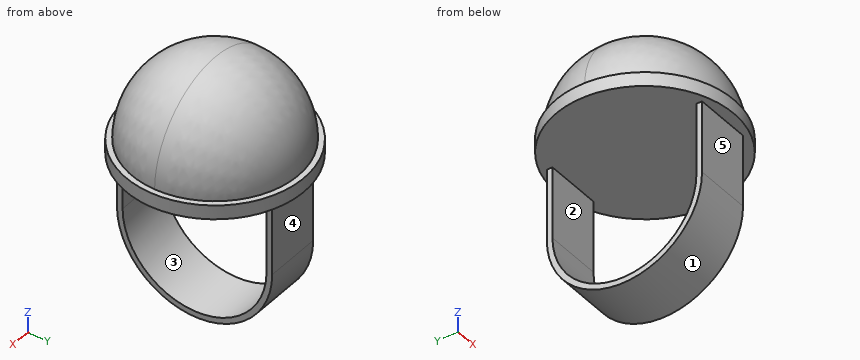
from build123d import *

# Parameters (mm, degrees)
F1_ANGLE = 180
F2_R     = 31.5
F3_DEPTH = 5
F4_W     = 20
F4_H     = 2
F5_DEPTH = 25.5
F6_W     = 20
F6_H     = 2
F7_ANGLE = 180


with BuildPart() as f1:
    # F0 (on Top) → F1 (revolve)
    with BuildSketch(Plane.XY):
        with BuildLine():
            ThreePointArc((0, -29.5), (20.85965, -20.85965), (29.5, 0))
            ThreePointArc((29.5, 0), (20.85965, 20.85965), (0, 29.5))
            Line((0, 29.5), (0, -29.5))
        make_face()
    revolve(axis=Axis((0, 0, 0), (0, -1, 0)), revolution_arc=F1_ANGLE)

    # F2 (on face) → F3 (join)
    with BuildSketch(Plane(origin=(0, 0, 0), x_dir=(1, 0, 0), z_dir=(0, 0, -1))):
        Circle(F2_R)
    extrude(amount=F3_DEPTH)

    # F4 (on face) → F5 (join)
    with BuildSketch(Plane(origin=(0, 0, -5), x_dir=(1, 0, 0), z_dir=(0, 0, -1))):
        with Locations((0, 26.5)):
            Rectangle(F4_W, F4_H)
        with Locations((0, -26.5)):
            Rectangle(F4_W, F4_H)
    extrude(amount=F5_DEPTH)

    # F6 (on face) → F7 (revolve)
    with BuildSketch(Plane(origin=(0, 0, -30.5), x_dir=(1, 0, 0), z_dir=(0, 0, -1))):
        with Locations((0, 26.5)):
            Rectangle(F6_W, F6_H)
    revolve(axis=Axis((7.741019, 0, -30.5), (1, 0, 0)), revolution_arc=F7_ANGLE)


solid = f1.part
Read the model definition and answer for the solid it produces. Units are mm, in the model's axes. Face numbers are marked on the shaded views. A direction names the side the tool comes from. Coordinates: 2 decimals unless noted, no trailing zeros. Loops run counter-clockwise (first coordinate to the right, second up) from the corner with the lowest first, then second, coordinate; pieces in that order, holes last.
Q1. Each of these flat-tipped pins is pushed along its axis until it touches: pin 1 Ø12 at (x, z) = (-9, -25.5) entering from -Y; pin 2 Ø6 at (x, z) = (19, 11.5) entering from -Y; pin 3 Ø1 at (x, y) = (-8, -4.5) entering from -Z. Where does it stop, or does it pass through?
Q2. Which of the six approach directions +Z, -Z, +X, -X, +Y, -Y give full straight-line access (tool end or side, diameter ignored) to the marked faces 1 and 2?
Q3. The part is cut by section A-A on z = -11. Write down the section's boundary in (x, y).
Q4. The part is cut by section B-B on z = -34. Write down the section's boundary in (x, y), and give its area (3 significant figures).
Q5. The mould has two halves that part along Y. Classify the marked faces 3, 4 and 5: +Y half, -Y half, draft (parallel to the pull), parting line (faces both ways), or undercut.
Q6. Consider probe 1 along Z at (x, y) = (1.5, 4.5); probe 2 along Z at (x, y) = (16.5, -25); probe 3 along Z at (x, y) = (15, -9). Determine where each line is inside the solid, lowest interval first.
Results below:
1. pin 1: stops at y = -27.5
1. pin 2: stops at y = -22.39
1. pin 3: stops at z = -57.71
2. face 1: -Z, +X, -X
2. face 2: +X, -X
3. outline: (-10, -27.5) - (10, -27.5) - (10, -25.5) - (-10, -25.5) - close; (-10, 25.5) - (10, 25.5) - (10, 27.5) - (-10, 27.5) - close
4. outline: (-10, -27.28) - (10, -27.28) - (10, -25.26) - (-10, -25.26) - close; (-10, 25.26) - (10, 25.26) - (10, 27.28) - (-10, 27.28) - close
4. area: 80.7 mm2
5. face 3: undercut
5. face 4: +Y half
5. face 5: -Y half
6. probe 1: z = -57.63 to -55.6, -5 to 29.12
6. probe 2: z = -5 to 0
6. probe 3: z = -5 to 23.75
